Can you work these out from the drawing? Everything is in mm from the part's minimum corner. Round coordinates to 2 decimals unless told otherwise and drop trailing zeros. Order: outer loops, then holes, each group sorted by start corner. A loop starts at its lowest first (then second) coordinate and runs counter-clockwise, first axis right, second up. Notation, with made-up numbers: (15.5, 55.5) -> (27.5, 55.5) arc R16 cw to (27.5, 74.5) -> close; hole circle Ø3 at (87.25, 72.5). An arc over 180 degrees is marked (long way). One line per item, written item: value.
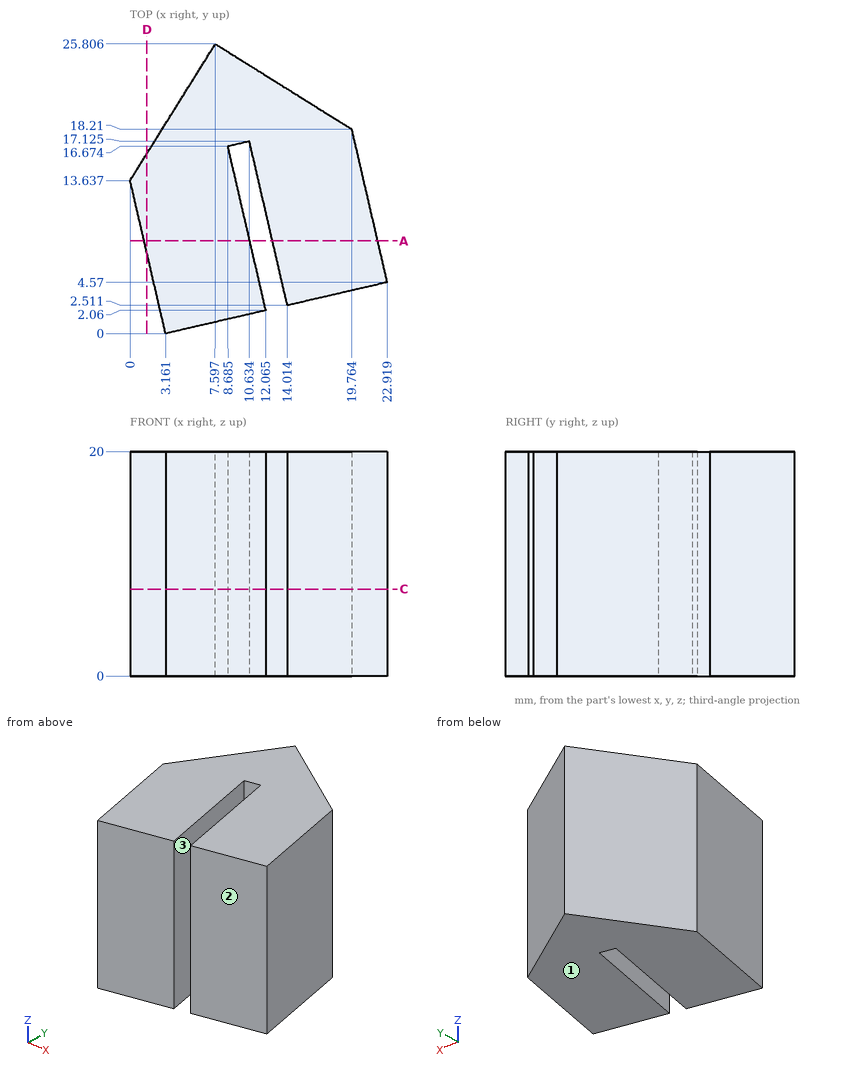
Q1. I want a section at A-A on y = 8.25. Write out the boundary of the cut face in (x, z).
Answers:
outline: (1.25, 0) -> (10.63, 0) -> (10.63, 20) -> (1.25, 20) -> close; (12.69, 0) -> (22.07, 0) -> (22.07, 20) -> (12.69, 20) -> close
Q2. I want a section at D-D on x = 1.5. Write out the boundary of the cut face in (y, z) (1 decimal).
Answers:
outline: (7.2, 0) -> (16, 0) -> (16, 20) -> (7.2, 20) -> close
Q3. I want a section at C-C on z = 7.75. Write out the boundary of the cut face in (x, y) (1 decimal).
Answers:
outline: (0, 13.6) -> (3.2, 0) -> (12.1, 2.1) -> (8.7, 16.7) -> (10.6, 17.1) -> (14, 2.5) -> (22.9, 4.6) -> (19.8, 18.2) -> (7.6, 25.8) -> close
Q4. If we mould it in two halves opening along Y, with no side actions, what happens to the marked faces 1, 2 and 3? For each: pulls with the +Y half, pulls with the -Y half, needs draft (parallel to the pull), parting line crosses it, or undercut.
Answers:
face 1: needs draft
face 2: pulls with the -Y half
face 3: undercut
Q5. For P1, Ø10, axis at x = 16.5, z = 17, coming from the +Y side; P2, Ø5, axis at x = 10.5, z = 14.5, coming from the +Y side (1 decimal), each with a flat end and sliding along its axis, tell me the tip position at first contact or that it passes through.
Answers:
P1: y = 23.37
P2: y = 25.6
Q6. I need wall thicknesses on line 1 along X through (y, z) = (10, 17.25); line 2 along X through (y, z) = (16.5, 16.5) (1 decimal); line 3 along Y through (x, z) = (16.5, 1.5) (1 decimal). Which ranges of each line are inside material? Lowest first, please.
Answers:
line 1: 0.84 to 10.23, 12.28 to 21.66
line 2: 1.8 to 8.7, 10.8 to 20.2
line 3: 3.1 to 20.2
